Part model, mm, in its own coordinate system. Face numbers are marked on the shaded views. A direction names the side the tool comes from. Give positions to 0.01 mm unless a question says otherwise; leave off trailing zeros. Write each loop counter-clockwise with the first axis right and the second up, starting at its lowest first coordinate (ties: lowest second). Pieces come first, ordered by that corner, then holes.
```python
from build123d import *

# Parameters (mm, degrees)
F1_DEPTH = 10
F2_R     = 1.4
F3_DEPTH = 25
F4_R     = 4.99999


# Not quite as in the source:
# - a fillet or chamfer is up to 0.001 mm smaller than in the source, because OpenCascade refuses the exact size


with BuildPart() as f1:
    # F0 (on Top) → F1 (new body)
    with BuildSketch(Plane.XY):
        with BuildLine():
            ThreePointArc((-3.5, 0), (0, 3.5), (3.5, 0))
            Line((3.5, 0), (3.5, -3.5))
            Line((3.5, -3.5), (13.5, -3.5))
            Line((13.5, -3.5), (13.5, -2))
            Line((13.5, -2), (6, -2))
            Line((6, -2), (6, 0))
            ThreePointArc((6, 0), (0, 6), (-6, 0))
            Line((-6, 0), (-6, -2))
            Line((-6, -2), (-13.5, -2))
            Line((-13.5, -2), (-13.5, -3.5))
            Line((-13.5, -3.5), (-3.5, -3.5))
            Line((-3.5, -3.5), (-3.5, 0))
        make_face()
    extrude(amount=F1_DEPTH)

    # F2 (on face) → F3 (cut)
    with BuildSketch(Plane(origin=(0, -2, 0), x_dir=(-1, 0, 0), z_dir=(0, 1, 0))):
        with Locations((9.75, 5)):
            Circle(F2_R)
        with Locations((-9.75, 5)):
            Circle(F2_R)
    extrude(amount=-F3_DEPTH, mode=Mode.SUBTRACT)

    # F4 (radius 5 in the source; OpenCascade refuses exactly that, so slightly less here)
    f4_edges = [f1.edges().sort_by_distance(p)[0] for p in [
        (-13.5, -2.75, 10),
        (13.5, -2.75, 10),
        (-13.5, -2.75, 0),
        (13.5, -2.75, 0),
    ]]
    fillet(f4_edges, radius=F4_R)


solid = f1.part
```
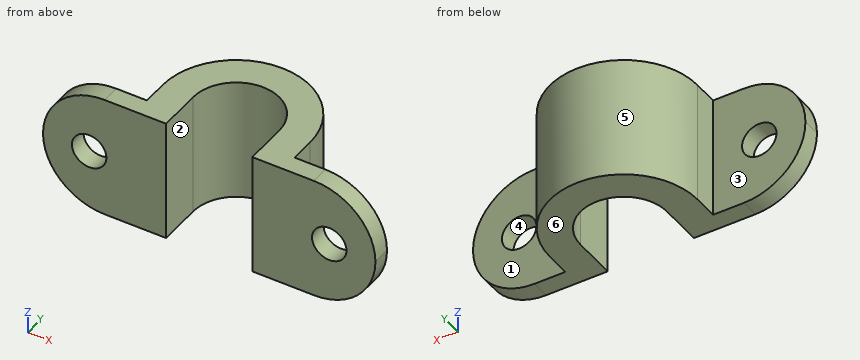
1) Saw through at C-C, the plane x = 9. Write the cut outline in (y, z).
Answers follow:
outline: (-3.5, 0.03) - (-2, 0.03) - (-2, 3.82) - (-3.5, 3.82) - close; (-3.5, 6.18) - (-2, 6.18) - (-2, 9.97) - (-3.5, 9.97) - close
2) Wall check: L1, parallel to X at y = -0.25, z = 6.25; L2, parallel to X at y = -3, z = 3.75; L3, parallel to Z at x = -9.75, y = -3. Give the ranges that are in metal, low to high.
Answers follow:
L1: x = -6 to -3.5, 3.5 to 6
L2: x = -13.34 to -10.38, -9.12 to -3.5, 3.5 to 9.12, 10.38 to 13.34
L3: z = 0.16 to 3.6, 6.4 to 9.84
3) 3-axis set-ups, long thin cutter, end or side, ignore diameter. For the marked faces 1, 2 and 3: which of +Z, -Z, +X, -X, +Y, -Y reach the whole face in a straight line?
Answers follow:
face 1: +Z, -Z, +X, +Y
face 2: +Z, -Z, -Y
face 3: +Z, -Z, -X, +Y
4) Saw through at B-B, the plane z = 8. Write the cut outline in (x, y), then the cut area to 3 significant figures.
Answers follow:
outline: (-12.5, -3.5) - (-3.5, -3.5) - (-3.5, 0) arc R3.5 cw to (3.5, 0) - (3.5, -3.5) - (12.5, -3.5) - (12.5, -2) - (6, -2) - (6, 0) arc R6 ccw to (-6, 0) - (-6, -2) - (-12.5, -2) - close
area: 74.3 mm2
5) Saw through at D-D, the plane z = 4.5. Write the cut outline in (x, y), then the cut area to 3 significant figures.
Answers follow:
outline: (-13.47, -3.5) - (-11.06, -3.5) - (-11.06, -2) - (-13.47, -2) - close; (-8.44, -3.5) - (-3.5, -3.5) - (-3.5, 0) arc R3.5 cw to (3.5, 0) - (3.5, -3.5) - (8.44, -3.5) - (8.44, -2) - (6, -2) - (6, 0) arc R6 ccw to (-6, 0) - (-6, -2) - (-8.44, -2) - close; (11.06, -3.5) - (13.47, -3.5) - (13.47, -2) - (11.06, -2) - close
area: 69.4 mm2
6) Pin check, flat tips, straight feed: pin 1 Ø0.6 at (y, z) = (-1, 4.5) entering from -X; pin 2 Ø1.5 at (y, z) = (2, 5.5) entering from -X; pin 3 Ø1.6 at (y, z) = (-1.5, 3.5) entering from +X; pin 4 Ø1.7 at (x, z) = (-9.75, 5) entering from -Y. Stop position of each tip, or through.
Answers follow:
pin 1: stops at x = -6
pin 2: stops at x = -5.87
pin 3: stops at x = 13.42
pin 4: passes through
7) Saw through at A-A, the plane y = -0.5. Write the cut outline in (x, z).
Answers follow:
outline: (-6, 0) - (-3.5, 0) - (-3.5, 10) - (-6, 10) - close; (3.5, 0) - (6, 0) - (6, 10) - (3.5, 10) - close
8) Two-plate mould, pull along Z, no slides. Class the marked faces 4, 5 and 6: +Z half, -Z half, draft (parallel to the pull), parting line (faces both ways), or undercut.
Answers follow:
face 4: undercut
face 5: draft
face 6: -Z half
